```python
from build123d import *

# Parameters (mm, degrees)
SKETCH2_R          = 6
CUT_EXTRUDE1_DEPTH = 11
CIRPATTERN1_COUNT  = 16


with BuildPart() as part:
    # Sketch1 → Revolve1 (revolve)
    with BuildSketch(Plane.XY):
        with BuildLine():
            Line((200, 0), (200, 10))
            Line((200, 10), (165, 10))
            Line((165, 10), (165, 30))
            ThreePointArc((165, 30), (156.213203436, 51.213203436), (135, 60))
            Line((135, 60), (85, 60))
            Line((85, 60), (85, 75))
            Line((85, 75), (50, 75))
            Line((50, 75), (50, 65))
            Line((50, 65), (75, 65))
            Line((75, 65), (75, 50))
            Line((75, 50), (135, 50))
            ThreePointArc((135, 50), (149.142135624, 44.142135624), (155, 30))
            Line((155, 30), (155, 0))
            Line((155, 0), (200, 0))
        make_face()
    revolve(axis=Axis((0, 0, 0), (0, 1, 0)))

    # Sketch2 → Cut-Extrude1 (cut, through all)
    with BuildSketch(Plane(origin=(0, 10, 0), x_dir=(1, 0, 0), z_dir=(0, 1, 0))):
        with Locations((182, 0)):
            Circle(SKETCH2_R)
    cut_extrude1 = extrude(amount=-CUT_EXTRUDE1_DEPTH, mode=Mode.SUBTRACT)

    # CirPattern1: Cut-Extrude1 ×16 about axis
    cirpattern1_axis = Axis((0, 0, 0), (0, 1, 0))
    for i in range(1, CIRPATTERN1_COUNT):
        add(cut_extrude1.rotate(cirpattern1_axis, i * 360 / CIRPATTERN1_COUNT), mode=Mode.SUBTRACT)


solid = part.part
```
Check sheet for the modelled part. Datum: model origin and axes. Units: mm. A direction names the side the tool comes from. Round coordinates to 2 decimals unless told otherwise and drop trailing zeros. Loops run counter-clockwise (first coordinate to the right, second up) from the corner with the lowest first, then second, coordinate; pieces in that order, holes last. Notation, with made-up numbers: M 59.5,51.25 L 109.5,51.25 A27 cw 109.5,90.25 Z; hole C 18,31 d7. An arc over 180 degrees is marked long. Answer as a JSON object with one key per item and string values.
1. Section check C-C (y = 19.5). Record the boundary of the cut face in (x, z).
Reply:
{"outline": "C 0,0 d330; hole C 0,0 d310"}
2. Mould release check, pull along X, two halves, no side actions. Record for faces 4 (the flat face through (-31, 10, -164)), 5 (the cylindrical face through (-35.769, 20.14, 161.076)), 6 (the cylindrical face through (169.19, 5.07, -75.557)), 7 (the cylindrical face through (-169.19, 5.07, 75.557)): pulls with the +X half, pulls with the -X half, needs draft (parallel to the pull), parting line crosses it, or undercut.
Reply:
{"face 4": "needs draft", "face 5": "parting line crosses it", "face 6": "undercut", "face 7": "undercut"}
3. Gauge pin test, flat ends, axial feed: P1, Ø12, axis at y = 38.5, z = -106, coming from the +X side; P2, Ø4, axis at x = 53, y = 18.5, coming from the +Z side; P3, Ø12, axis at x = -65, y = 24, coming from the -Z side; P4, Ø9.5, axis at x = -168.15, z = 69.65, coming from the -Y side. Record the tip position at first contact, or that the pin passes through.
Reply:
{"P1": "stops at x = 130.08", "P2": "stops at z = 156.92", "P3": "stops at z = -154.09", "P4": "passes through"}
4. Scan lines: line 1 (Z direction, x = 0, y = 71); line 2 (X direction, y = 11.75, z = 0); line 3 (Y direction, x = 180, z = -62.5). Record each from-to range of solid material in increasing order.
Reply:
{"line 1": "z = -85 to -50, 50 to 85", "line 2": "x = -165 to -155, 155 to 165", "line 3": "y = 0 to 10"}
5. Section check D-D (x = -182). Record the boundary of the cut face in (y, z).
Reply:
{"outline": "M 0,-82.92 L 10,-82.92 L 10,-6 L 0,-6 Z; M 0,6 L 10,6 L 10,82.92 L 0,82.92 Z"}
6. Section check A-A (z = -182). Record the boundary of the cut face in (x, y).
Reply:
{"outline": "M -82.92,0 L -6,0 L -6,10 L -82.92,10 Z; M 6,0 L 82.92,0 L 82.92,10 L 6,10 Z"}
7. Section check B-B (x = 0). State how many separate pieces and enclosed holes the cut face has, plus the area to 3 significant figures.
Reply:
{"separate pieces": "4", "enclosed holes": "0", "area": "3,850 mm²"}
8. Access from +Z, -Z, +X, -X, +Y, -Y to the whole of each face (thin tool, end or side, straight path). Record for faces 1 (the cylindrical face through (-67.453, 67.605, 51.721)), 2 (the cylindrical face through (127.908, 5.07, -122.745)), 3 (the flat face through (-58, 50, 58)).
Reply:
{"face 1": "+Y", "face 2": "+Y, -Y", "face 3": "-Y"}
